from build123d import *

# Parameters (mm, degrees)
F0_R     = 15
F1_DEPTH = 300
F2_R     = 5
F3_DEPTH = 25
F4_R     = 5
F5_DEPTH = 25


with BuildPart() as f1:
    # F0 (on Right) → F1 (new body)
    with BuildSketch(Plane.YZ):
        Circle(F0_R)
    extrude(amount=F1_DEPTH)

    # F2 (on face) → F3 (join)
    with BuildSketch(Plane(origin=(0, 0, 0), x_dir=(0, -1, 0), z_dir=(-1, 0, 0))):
        Circle(F2_R)
    extrude(amount=F3_DEPTH)

    # F4 (on face) → F5 (join)
    with BuildSketch(Plane.YZ.offset(300)):
        Circle(F4_R)
    extrude(amount=F5_DEPTH)


solid = f1.part
Input: part model. Units: mm. Frame: model coordinates. A direction names the side the tool comes from. Coordinates: 2 decimals unless noted, no trailing zeros. Loops run counter-clockwise (first coordinate to the right, second up) from the corner with the lowest first, then second, coordinate; pieces in that order, holes last. Notation, with made-up numbers: (44.25, -21) -> (76.25, -21) arc R34 ccw to (76.25, 16) -> close; hole circle Ø10 at (-22.75, 83). An arc over 180 degrees is marked (long way). Write each question's results on one line, items separated by ' | '. Start each with the question number.
Q1. Pin query (flat end, axial travel): pin 1 (1 mm diameter, centred on x = 264.5, y = -7.5, fed in from +Z); pin 2 (1 mm diameter, centred on x = 36, z = -9.5, fed in from +Y); pin 3 (4 mm diameter, centred on y = 5, z = -8, fed in from -X). Return the tip coordinate at first contact, or that it passes through.
Q2. Ray query, line 1 (X direction, y = -6.5, z = 9.25); line 2 (Z direction, x = 78.5, y = 7.25); line 3 (Y direction, x = 233.5, z = -5.5). Return the intervals inside material, ascending. Write a range as from..to.
Q3. Section A-A, the plane z = 0. Return the cut outline in (x, y), plus the area to 3 significant figures.
Q4. Reachability of faces 1 (the flat face through (300, -4, 4)), 2 (the cylindrical face through (-12.32, 1.08, -4.88)), 3 (the flat face through (325, 0, 0)) from +Z, -Z, +X, -X, +Y, -Y: full face, straight path, thin tool, end or side. Return the list, or none.
Q5. Section C-C, the plane x = 9.5. Return the cut outline in (y, z).
Found:
1) pin 1: z = 13.27 | pin 2: y = 12 | pin 3: x = 0
2) line 1: 0..300 | line 2: -13.13..13.13 | line 3: -13.96..13.96
3) outline: (-25, -5) -> (0, -5) -> (0, -15) -> (300, -15) -> (300, -5) -> (325, -5) -> (325, 5) -> (300, 5) -> (300, 15) -> (0, 15) -> (0, 5) -> (-25, 5) -> close | area: 9,500 mm2
4) face 1: +X | face 2: -X | face 3: +Z, -Z, +X, +Y, -Y
5) outline: circle Ø30 at (0, 0)
